```python
from build123d import *

# Parameters (mm, degrees)
F1_DEPTH = 53.848
F2_R     = 8.4604896976
F3_DEPTH = 64.262
F4_R     = 5.08


with BuildPart() as f1:
    # F0 (on Top) → F1 (new body)
    with BuildSketch(Plane.XY):
        Polygon((24.7506033629, 22.1318155527), (-55.6636229157, 22.1318155527), (-60.4034848511, -28.4259710461), (24.7506033629, -32.2828106582), align=None)
    extrude(amount=F1_DEPTH)

    # F2 (on face) → F3 (cut)
    with BuildSketch(Plane(origin=(-1.4085054524, -31.0979998146, 0), x_dir=(0.9989758712, -0.045246092, 0), z_dir=(-0.045246092, -0.9989758712, 0))):
        with Locations((-13.3521184325, 30.6290015578)):
            Circle(F2_R)
    extrude(amount=-F3_DEPTH, mode=Mode.SUBTRACT)

    # F4
    f4_edges = [f1.edges().sort_by_distance(p)[0] for p in [
        (-60.403485, -28.425971, 26.924),
        (-17.826441, -30.354391, 0),
        (-17.826441, -30.354391, 53.848),
        (24.750603, -32.282811, 26.924),
        (-23.198775, -30.111065, 30.629002),
        (-58.033554, -3.147078, 53.848),
        (-55.663623, 22.131816, 26.924),
        (24.750603, -5.075498, 53.848),
    ]]
    fillet(f4_edges, radius=F4_R)


solid = f1.part
```
For this review, take the finished solid that the model builds, in its own axes (mm). Round coordinates to 2 decimals unless told otherwise and drop trailing zeros. Write each loop counter-clockwise with the first axis right and the second up, starting at its lowest first coordinate (ties: lowest second). Pieces come first, ordered by that corner, then holes. Notation, with made-up numbers: (9, 9.5) - (23, 9.5) arc R17 ccw to (23, 39.5) - close; hole circle Ø3 at (69, -39.5). An arc over 180 degrees is marked (long way). Write each question's results on one line, items separated by ' | '.
Item 1: For pin 1 (8 mm diameter, centred on y = -10.5, z = 13.5, fed in from -X); pin 2 (10 mm diameter, centred on x = 9.5, z = 7.5, fed in from -Y), all flat-tipped, find the tip position at first contact; note any pin that passes through.
Calculated:
pin 1: stops at x = -59.1 | pin 2: stops at y = -31.82
Item 2: Draft analysis for pull direction Z (two halves, no side actions). For faces 1 (the face through (-58.72, -26.88, 24.73)), 2 (the face through (-15.28, -1.7, 22.37)), 3 (the face through (-17.157, -28.856, 1.449)), 4 (the face through (23.3, -2.07, 52.32)), state which applies: pulls with the +Z half, pulls with the -Z half, needs draft (parallel to the pull), parting line crosses it, or undercut.
Calculated:
face 1: needs draft | face 2: undercut | face 3: pulls with the -Z half | face 4: pulls with the +Z half
Item 3: Take a section at A-A on z = 47. State the section outline as (x, y) points.
Calculated:
outline: (-59.91, -23.12) arc R5.08 ccw to (-55.08, -28.67) - (19.44, -32.04) arc R5.08 ccw to (24.75, -26.97) - (24.75, 22.13) - (-51.04, 22.13) arc R5.08 ccw to (-56.1, 17.53) - close
Item 4: To check wall thickness, follow line 1 along Z through (x, y) = (-14.5, -14.5); line 2 along X through (y, z) = (-7.5, 25); line 3 along Z through (x, y) = (-7.5, -14). State the ranges of each line that lie inside material, in increasing order. Write a range as from..to.
Calculated:
line 1: z = 0..22.18, 39.08..53.85 | line 2: x = -58.44..-20.03, -7.38..24.75 | line 3: z = 0..25.21, 36.05..53.85
